Autodesk Inventor part; units mm, degrees
ref_plane "YZ Plane" through (0, 0, 0) normal (1, 0, 0) x (0, 1, 0)
ref_plane "XZ Plane" through (0, 0, 0) normal (0, 1, 0) x (-1, 0, 0)
ref_plane "XY Plane" through (0, 0, 0) normal (0, 0, 1) x (1, 0, 0)
sketch "Sketch1" plane through (0, 0, 0) normal (0, 1, 0) x (-1, 0, 0)
  circle A0 centre (0, 0) radius 7
  circle A1 centre (0, 0) radius 10
  line L0 (0, 11.563) -> (0, -13.4764)
  point P0 (0, -7)
  point P1 (0, -10)
  point P2 (0, 10)
  point P3 (0, 7)
  dimension "d0" = 14
  dimension "d1" = 20
extrude "Extrusion1" add sketch "Sketch1" along normal blind 25 contours A0 L0 A1 picked at (8.8579, -1.261)
sketch "Sketch2" plane through (0, 25, 0) normal (0, 1, 0) x (1, 0, 0)
  arc A0 (0, 7) -> (0, -7) centre (0, 0) ccw
  point P0 (-7, 0)
ref_plane "Work Plane1" through (-7, 25, 0) normal (1, 0, 0) x (0, 0, -1)
sketch "Sketch3" plane through (-7, 25, 0) normal (1, 0, 0) x (0, 0, -1)
  line L0 (10, 0) -> (-10, 0)
  line L1 (0, 0) -> (0, -5)
  line L2 (0, -5) -> (0, -6.25)
  line L3 (0, -5) -> (1.0825, -5.625)
  line L4 (1.0825, -5.625) -> (1.0825, -6.875)
  line L5 (1.0825, -6.875) -> (0, -7.5)
  line L6 (0, -7.5) -> (-1.0825, -6.875)
  line L7 (-1.0825, -6.875) -> (-1.0825, -5.625)
  line L8 (-1.0825, -5.625) -> (0, -5)
  line L9 (0, -6.25) -> (0, -21.25)
  line L10 (0, -21.25) -> (0, -22.5)
  line L11 (0, -22.5) -> (-1.0825, -21.875)
  line L12 (-1.0825, -21.875) -> (-1.0825, -20.625)
  line L13 (-1.0825, -20.625) -> (0, -20)
  line L14 (0, -20) -> (1.0825, -20.625)
  line L15 (1.0825, -20.625) -> (1.0825, -21.875)
  line L16 (1.0825, -21.875) -> (0, -22.5)
  point P0 (0, -25)
  dimension "d4" = 5
  dimension "d5" = 1.25
  dimension "d6" = 15
  dimension "d7" = 1.25
extrude "Extrusion2" add sketch "Sketch3" along normal blind 2
sketch "Sketch4" plane through (-7, 25, 0) normal (1, 0, 0) x (0, 0, -1)
  line L0 (0, -25) -> (0, 0)
  line L1 (-7, 0) -> (7, 0)
  line L2 (0, -12.5) -> (-3, -12.5)
  circle A0 centre (0, -12.5) radius 3
  dimension "d10" = 3
extrude "Extrusion3" add sketch "Sketch4" against normal blind 30
sketch "Sketch5" plane through (0, 0, 0) normal (0, -1, 0) x (1, 0, 0)
  line L0 (-37, 3) -> (-37, -3)
  line L1 (-37, -3) -> (-34, -3)
  line L2 (-9.5394, -3) -> (-37, -3)
  line L3 (-34, -3) -> (-34, 0)
  line L4 (-34, 0) -> (-34, -1.5)
  line L5 (-34, -1.5) -> (-33, -1.5)
  line L6 (-33, -1.5) -> (-33, -3)
  line L7 (-33, -3) -> (-34.954, -5.8523)
  line L8 (-34.954, -5.8523) -> (-37, -3)
  point P0 (0, 0)
  point P1 (-9.5394, 3)
  dimension "d13" = 3
  dimension "d14" = 1
extrude "Extrusion4" cut sketch "Sketch5" against normal through all
sketch "Sketch6" plane through (0, 0, 0) normal (0, -1, 0) x (1, 0, 0)
  point P0 (0, 0)
properties part number "medidor_torque_palanca"
Here's how the part is built. I have some questions about the finished solid (model axes, mm). A direction names the side the tool comes from. Coordinates: 2 decimals unless noted, no trailing zeros. Order: outer loops, then holes, each group sorted by start corner. A loop starts at its lowest first (then second) coordinate and runs counter-clockwise, first axis right, second up.
Item 1: I need wall thicknesses on line 1 (Y direction, x = -11.5, z = 0); line 2 (Z direction, x = -3, y = 17.75); line 3 (X direction, y = 12.75, z = -8.75). Which ranges of each line are inside material? Lowest first, please.
Result sheet:
line 1: y = 9.5 to 15.5
line 2: z = -9.54 to -6.32, 6.32 to 9.54
line 3: x = -4.84 to 0
Item 2: If we section it at C-C on x = -30.5: List the corners of the cut face in (y, z) for me.
Result sheet:
outline: circle Ø6 at (12.5, 0)
Item 3: If we mould it in two halves opening along Y, with no side actions, what happens to faces 1 (the face through (-6.014, 19.683, 0.549)), 2 (the face through (-33, 12, -2)), 3 (the face through (-6.014, 4.692, -0.534))? For each: +Y half, -Y half, draft (parallel to the pull), parting line (faces both ways), or undercut.
Result sheet:
face 1: +Y half
face 2: draft
face 3: undercut
Item 4: For faces 4 (the face through (-6.014, 2.808, 0.534)), 5 (the face through (-6, 4, -1.082)), 6 (the face through (-6.014, 17.817, -0.549)), which set-ups out of +Z, -Z, +X, -X, +Y, -Y let a thin tool reach every point of the face, with its end or its side?
Result sheet:
face 4: +X, -Y
face 5: +X, +Y, -Y
face 6: +X
Item 5: If we section it at D-D on z = 1.5: List the corners of the cut face in (x, y) for me, plus the area to 3 significant figures.
Result sheet:
outline: (-37, 9.9) - (-9.89, 9.9) - (-9.89, 0) - (-6.84, 0) - (-6.84, 25) - (-9.89, 25) - (-9.89, 15.1) - (-37, 15.1) - close
area: 217 mm2
Item 6: If we section it at B-B on y = 12.5: List the corners of the cut face in (x, z) for me, plus the area to 3 significant figures.
Result sheet:
outline: (-37, -3) - (-34, -3) - (-34, -1.5) - (-33, -1.5) - (-33, -3) - (-9.54, -3) arc R10 ccw to (0, -10) - (0, -7) arc R7 cw to (0, 7) - (0, 10) arc R10 ccw to (-9.54, 3) - (-37, 3) - close
area: 242 mm2
Item 7: If we section it at A-A on z = -2.5: List the corners of the cut face in (x, y) for me, plus the area to 3 significant figures.
Result sheet:
outline: (-37, 10.84) - (-34, 10.84) - (-34, 14.16) - (-37, 14.16) - close; (-33, 10.84) - (-9.68, 10.84) - (-9.68, 0) - (-6.54, 0) - (-6.54, 25) - (-9.68, 25) - (-9.68, 14.16) - (-33, 14.16) - close
area: 166 mm2
Item 8: For P1, Ø2, axis at x = -7, y = 10.5, coming from the +Z side; P2, Ø1, axis at y = 4, z = 5, coming from the +X side; P3, Ø0.6, axis at x = -5.5, y = 18.5, coming from the -Z side; P4, Ø5, axis at x = -6, z = 3, coming from the -Y side, each with a flat end and sliding along its axis, tell me the tip position at first contact or that it passes through.
Result sheet:
P1: stops at z = 8
P2: stops at x = -4.33
P3: stops at z = -8.54
P4: stops at y = 0
